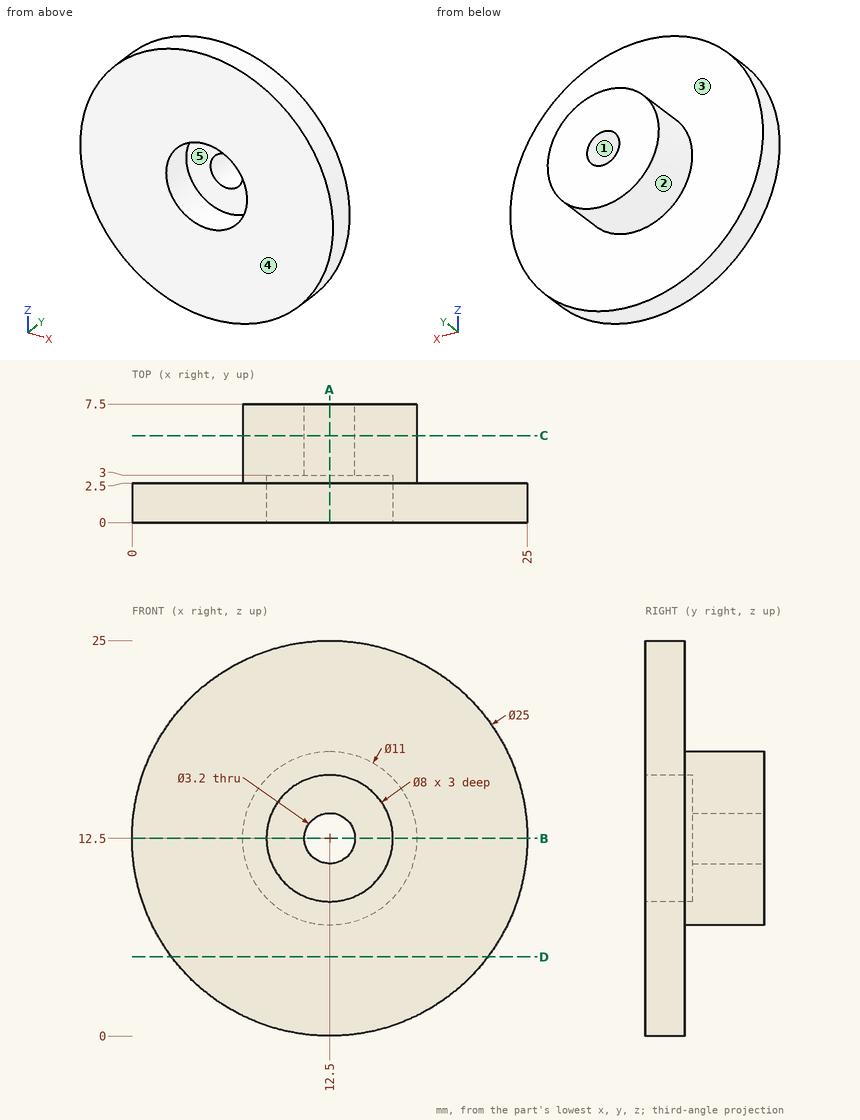
Here's the drawing with two shaded views (mm, measured from the low corner). I have some questions. A direction names the side the tool comes from. Coordinates: 2 decimals unless noted, no trailing zeros. Loops run counter-clockwise (first coordinate to the right, second up) from the corner with the lowest first, then second, coordinate; pieces in that order, holes last. Notation, with made-up numbers: M -26,-0.75 L 13,-0.75 A25 cw 13,26.25 Z; hole C -25.5,-4 d9. An arc over 180 degrees is marked long. Return JSON: item names as keys, results as strings. Group by question number.
Item 1: Imagine slicing it at B-B (z = 12.5). Please give me the cut outline in (x, y), and give its area (3 significant figures).
Item 2: Imagine slicing it at C-C (y = 5.5). Please give me the cut outline in (x, z).
Item 3: Imagine slicing it at A-A (x = 12.5). Please give me the cut outline in (y, z).
Item 4: Thinking about a two-plate mould opening in Z: for the marked faces 1, 2 and 3, which applies, released by +Z, released by -Z, zero draft, split by the parting line, or undercut?
Item 5: Imagine slicing it at D-D (z = 5). Please give me the cut outline in (x, y).
Item 6: I'm going to push flat-ended pins straight in: pin 1 Ø4 at (y, z) = (2.5, 16.5) entering from +X; pin 2 Ø1 at (x, y) = (12.5, 4) entering from +Z; pin 3 Ø1 at (x, y) = (20.5, 1) entering from -Z. Where does each tip first touch, or does it pass through?
Item 7: On a 3-axis mill with a long thin cutter (end or side, diameter ignored), from which of +Z, -Z, +X, -X, +Y, -Y can I reach the whole of each face in a straight line? I mean the marked faces 4 and 5. Say none if no direction works.
Item 8: If I drill on L1, parallel to Y at x = 14.5, z = 23.5; L2, parallel to X at y = 2, z = 9; L3, parallel to X at y = 2, z = 15.25, over which ranges is the centre line in solid material (lowest first)? Write a range as from..to.
Verdict:
{
 "1": {"outline": "M 0,0 L 8.5,0 L 8.5,3 L 10.9,3 L 10.9,7.5 L 7,7.5 L 7,2.5 L 0,2.5 Z; M 14.1,3 L 16.5,3 L 16.5,0 L 25,0 L 25,2.5 L 18,2.5 L 18,7.5 L 14.1,7.5 Z", "area": "79.1 mm^2"},
 "2": {"outline": "C 12.5,12.5 d11; hole C 12.5,12.5 d3.2"},
 "3": {"outline": "M 0,0 L 2.5,0 L 2.5,7 L 7.5,7 L 7.5,10.9 L 3,10.9 L 3,8.5 L 0,8.5 Z; M 0,16.5 L 3,16.5 L 3,14.1 L 7.5,14.1 L 7.5,18 L 2.5,18 L 2.5,25 L 0,25 Z"},
 "4": {"face 1": "undercut", "face 2": "split by the parting line", "face 3": "zero draft"},
 "5": {"outline": "M 2.5,0 L 22.5,0 L 22.5,2.5 L 2.5,2.5 Z"},
 "6": {"pin 1": "stops at x = 24.84", "pin 2": "stops at z = 18", "pin 3": "stops at z = 2.5"},
 "7": {"face 4": "+Z, -Z, +X, -X, -Y", "face 5": "-Y"},
 "8": {"L1": "y = 0..2.5", "L2": "x = 0.5..10.56, 14.44..24.5", "L3": "x = 0.31..9.6, 15.4..24.69"}
}
